Verification items for the finished model (mm, model axes). Give positions to 0.01 mm unless a question says otherwise; leave off trailing zeros. Loops run counter-clockwise (first coordinate to the right, second up) from the corner with the lowest first, then second, coordinate; pieces in that order, holes last. Notation, with made-up numbers: M 10,-17 L 68,-17 A4 cw 68,-13 Z; hole C 25,40.25 d1. An arc over 180 degrees is marked long. Answer in a Markdown table with one row per item.
```python
from build123d import *

# Parameters (mm, degrees)
SKETCH_1_W          = 60
SKETCH_1_H          = 30
BOARD_DEPTH         = 1.58
SKETCH_2_R          = 1.7
CUT_EXTRUDE_1_DEPTH = 1.58
SKETCH_3_R          = 1.7
CUT_EXTRUDE_2_DEPTH = 469.617644141
SKETCH_4_R          = 1.7
CUT_EXTRUDE_3_DEPTH = 469.617644141
SKETCH_5_R          = 1.7
CUT_EXTRUDE_4_DEPTH = 469.617644141
SKETCH_6_R          = 0.35
SKETCH_6_R_2        = 0.4
SKETCH_6_R_3        = 0.9
SKETCH_6_R_4        = 1.5
SKETCH_6_R_5        = 0.45
CUT_EXTRUDE_5_DEPTH = 469.617644141


with BuildPart() as part:
    # 草圖1 → Board (new body)
    with BuildSketch(Plane.XY):
        with Locations((330, 285)):
            Rectangle(SKETCH_1_W, SKETCH_1_H)
    extrude(amount=BOARD_DEPTH)

    # 草圖2 → 除料-伸長1 (cut)
    with BuildSketch(Plane.XY.offset(1.58)):
        with Locations((357, 297)):
            Circle(SKETCH_2_R)
    extrude(amount=-CUT_EXTRUDE_1_DEPTH, mode=Mode.SUBTRACT)

    # 草圖3 → 除料-伸長2 (cut, through all)
    with BuildSketch(Plane.XY.offset(1.58)):
        with Locations((357, 273)):
            Circle(SKETCH_3_R)
    extrude(amount=-CUT_EXTRUDE_2_DEPTH, mode=Mode.SUBTRACT)

    # 草圖4 → 除料-伸長3 (cut, through all)
    with BuildSketch(Plane.XY.offset(1.58)):
        with Locations((303, 273)):
            Circle(SKETCH_4_R)
    extrude(amount=-CUT_EXTRUDE_3_DEPTH, mode=Mode.SUBTRACT)

    # 草圖5 → 除料-伸長4 (cut, through all)
    with BuildSketch(Plane.XY.offset(1.58)):
        with Locations((303, 297)):
            Circle(SKETCH_5_R)
    extrude(amount=-CUT_EXTRUDE_4_DEPTH, mode=Mode.SUBTRACT)

    # 草圖6 → 除料-伸長5 (cut, through all)
    with BuildSketch(Plane.XY.offset(1.58)):
        with Locations((337, 296)):
            Circle(SKETCH_6_R)
        with Locations((328.99999, 296)):
            Circle(SKETCH_6_R)
        with Locations((335, 296)):
            Circle(SKETCH_6_R)
        with Locations((333, 296)):
            Circle(SKETCH_6_R)
        with Locations((331, 296)):
            Circle(SKETCH_6_R)
        with Locations((339, 296)):
            Circle(SKETCH_6_R)
        with Locations((310.8, 274)):
            Circle(SKETCH_6_R_2)
        with Locations((310.8, 279)):
            Circle(SKETCH_6_R_2)
        with Locations((352, 290)):
            Circle(SKETCH_6_R)
        with Locations((352, 288)):
            Circle(SKETCH_6_R)
        with Locations((352, 286)):
            Circle(SKETCH_6_R)
        with Locations((352, 282)):
            Circle(SKETCH_6_R)
        with Locations((352, 284)):
            Circle(SKETCH_6_R)
        with Locations((352, 280)):
            Circle(SKETCH_6_R)
        with Locations((309.9, 289)):
            Circle(SKETCH_6_R_3)
        with Locations((314.1, 289)):
            Circle(SKETCH_6_R_3)
        with Locations((309.9, 283.5)):
            Circle(SKETCH_6_R_3)
        with Locations((312, 296.3)):
            Circle(SKETCH_6_R_4)
        with Locations((314.1, 283.5)):
            Circle(SKETCH_6_R_3)
        with Locations((358, 290)):
            Circle(SKETCH_6_R)
        with Locations((358, 288)):
            Circle(SKETCH_6_R)
        with Locations((358, 286)):
            Circle(SKETCH_6_R)
        with Locations((358, 282)):
            Circle(SKETCH_6_R)
        with Locations((358, 284)):
            Circle(SKETCH_6_R)
        with Locations((358, 280)):
            Circle(SKETCH_6_R)
        with Locations((331.46, 274)):
            Circle(SKETCH_6_R_5)
        with Locations((336.54, 274)):
            Circle(SKETCH_6_R_5)
        with Locations((334, 274)):
            Circle(SKETCH_6_R_5)
        with Locations((343, 296)):
            Circle(SKETCH_6_R)
        with Locations((341, 296)):
            Circle(SKETCH_6_R)
        with Locations((345, 296)):
            Circle(SKETCH_6_R)
        with Locations((347, 296)):
            Circle(SKETCH_6_R)
        with Locations((349, 296)):
            Circle(SKETCH_6_R)
        with Locations((351, 296)):
            Circle(SKETCH_6_R)
        with Locations((319.46, 274)):
            Circle(SKETCH_6_R_5)
        with Locations((324.54, 274)):
            Circle(SKETCH_6_R_5)
        with Locations((322, 274)):
            Circle(SKETCH_6_R_5)
        with Locations((348.54, 274)):
            Circle(SKETCH_6_R_5)
        with Locations((346, 274)):
            Circle(SKETCH_6_R_5)
        with Locations((343.46, 274)):
            Circle(SKETCH_6_R_5)
    extrude(amount=-CUT_EXTRUDE_5_DEPTH, mode=Mode.SUBTRACT)


solid = part.part
```
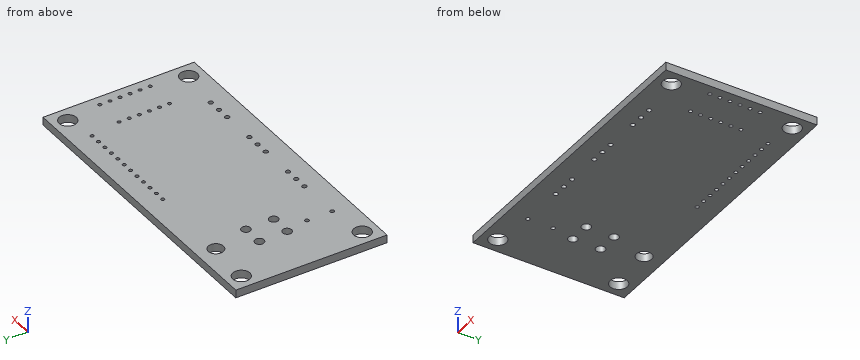
Item 1: Sectioned sample at B-B (y = 289). Record the cut outline in (x, z).
Reported:
| item | result |
|---|---|
| outline | M 300,0 L 309,0 L 309,1.58 L 300,1.58 Z; M 310.8,0 L 313.2,0 L 313.2,1.58 L 310.8,1.58 Z; M 315,0 L 360,0 L 360,1.58 L 315,1.58 Z |
Item 2: Scan lines: L1, parallel to X at y = 282, z = 1.1; L2, parallel to X at y = 273.25, z = 0.3; L3, parallel to Y at x = 346, z = 1. Record each from-to range of solid material in increasing order. Write a range as [from, to].
Reported:
| item | result |
|---|---|
| L1 | x = [300, 351.65], [352.35, 357.65], [358.35, 360] |
| L2 | x = [300, 301.32], [304.68, 355.32], [358.68, 360] |
| L3 | y = [270, 273.55], [274.45, 300] |
Item 3: Sectioned sample at D-D (z = 1.1). State how many separate pieces and enclosed holes the cut face has, and give its area (3 significant figures).
Reported:
| item | result |
|---|---|
| separate pieces | 1 |
| enclosed holes | 44 |
| area | 1,730 mm^2 |
Item 4: Sectioned sample at C-C (x = 312). Record the cut outline in (y, z), and give its area (3 significant figures).
Reported:
| item | result |
|---|---|
| outline | M 270,0 L 294.8,0 L 294.8,1.58 L 270,1.58 Z; M 297.8,0 L 300,0 L 300,1.58 L 297.8,1.58 Z |
| area | 42.7 mm^2 |
Item 5: Go/stop test with flat-tipped pins: pin 1 (3 mm diameter, centred on x = 314.1, y = 289, fed in from -Z); pin 2 (3 mm diameter, centred on x = 357, y = 297, fed in from -Z). Record where each tip stops, or that it passes through.
Reported:
| item | result |
|---|---|
| pin 1 | stops at z = 0 |
| pin 2 | passes through |
Item 6: Sectioned sample at A-A (x = 303). Record the cut outline in (y, z).
Reported:
| item | result |
|---|---|
| outline | M 270,0 L 271.3,0 L 271.3,1.58 L 270,1.58 Z; M 274.7,0 L 295.3,0 L 295.3,1.58 L 274.7,1.58 Z; M 298.7,0 L 300,0 L 300,1.58 L 298.7,1.58 Z |
